For this review, take the finished solid that the model builds, in its own axes (mm). Face numbers are marked on the shaded views. A direction names the side the tool comes from. Round coordinates to 2 decimals unless told otherwise and drop trailing zeros. Loops run counter-clockwise (first coordinate to the right, second up) from the corner with the lowest first, then second, coordinate; pieces in that order, holes last.
1) Wall thickness on L1, parallel to Z at x = -37, y = -20.95; L2, parallel to X at y = -1, z = 53; L3, parallel to Z at x = -10, y = 4: over which ranges is each line inside the solid? List them lowest first.
2) Mouldability with a two-part tool opening along X and no side actions: class the marked faces 6, 7 and 8 as pulls with the +X half, pulls with the -X half, needs draft (parallel to the pull), parting line crosses it, or undercut.
3) Take a section at B-B (z = 60). State the section outline as (x, y) points.
4) Take a section at D-D (x = -30). State the section outline as (y, z) points.
5) Take a section at C-C (x = 0). State the section outline as (y, z) points.
6) Take a section at A-A (x = 37). State the section outline as (y, z) points.
7) Tool access review of the marked faces 1, 2, 3, 4 and 5: name each direction out of +Z, -Z, +X, -X, +Y, -Y from which nothing blocks a thin tool from reaching the whole face with its end or side.
8) Insertion check: pin 1 (4.5 mm diameter, centred on x = -15.5, y = 0, fed in from -Z); pin 2 (2.5 mm diameter, centred on x = 20, z = 61, fed in from +Y); pin 3 (1.5 mm diameter, centred on x = -36.5, z = 30.5, fed in from +Y); pin 4 (8 mm diameter, centred on x = -2, y = 1, fed in from +Z). Each pin has a flat end and moves straight along its axis. Give the tip position at first contact, or say it passes through.
```python
from build123d import *

# Parameters (mm, degrees)
SKETCH3_R                      = 7.25
BOSS_EXTRUDE1_DEPTH            = 5
M3_CLEARANCE_HOLE1_D           = 3.4
M3_CLEARANCE_HOLE1_CSINK_D     = 3.45
M3_CLEARANCE_HOLE1_CSINK_ANGLE = 90
BOSS_EXTRUDE2_DEPTH            = 80
BOSS_EXTRUDE3_DEPTH            = 10
SKETCH16_R                     = 11
CUT_EXTRUDE1_DEPTH             = 7
CUT_EXTRUDE2_REACH             = 90
SKETCH17_R                     = 7
CHAMFER2_SIZE                  = 0.5
CHAMFER3_SIZE                  = 0.5
SKETCH18_W                     = 95
SKETCH18_H                     = 5.838314525
BOSS_EXTRUDE5_DEPTH            = 30
SKETCH21_W                     = 95
SKETCH21_H                     = 5
BOSS_EXTRUDE6_DEPTH            = 30
FILLET1_R                      = 5
M5_CLEARANCE_SLOT1_D           = 5.3


with BuildPart() as part:
    # Sketch3 → Boss-Extrude1 (new body)
    with BuildSketch(Plane.XY):
        with BuildLine():
            Line((22, 0), (22, -22))
            Line((22, -22), (-22, -22))
            Line((-22, -22), (-22, 0))
            ThreePointArc((-22, 0), (0, 22), (22, 0))
        make_face()
        with Locations((0, 7)):
            Circle(SKETCH3_R, mode=Mode.SUBTRACT)
    extrude(amount=BOSS_EXTRUDE1_DEPTH)

    # M3 Clearance Hole1 (through all)
    with Locations(Plane(origin=(0, 0, 0), x_dir=(-1, 0, 0), z_dir=(0, 0, -1))):
        with Locations((-15.5, 0), (15.5, 0), (7.75, 13.423393759), (-7.75, 13.423393759), (-7.75, -13.423393759), (7.75, -13.423393759)):
            CounterSinkHole(M3_CLEARANCE_HOLE1_D / 2, M3_CLEARANCE_HOLE1_CSINK_D / 2, counter_sink_angle=M3_CLEARANCE_HOLE1_CSINK_ANGLE)

    # Sketch7 → Boss-Extrude2 (add)
    with BuildSketch(Plane.XY.offset(5)):
        with BuildLine():
            Line((-19, 0), (-22, 0))
            Line((-22, 0), (-22, -22))
            Line((-22, -22), (22, -22))
            Line((22, -22), (22, 0))
            Line((22, 0), (19, 0))
            ThreePointArc((19, 0), (0, -19), (-19, 0))
        make_face()
    extrude(amount=BOSS_EXTRUDE2_DEPTH)

    # Sketch9 → Boss-Extrude3 (add)
    with BuildSketch(Plane.XY.offset(85)):
        with BuildLine():
            Line((22, 0), (22, -22))
            Line((22, -22), (-22, -22))
            Line((-22, -22), (-22, 0))
            ThreePointArc((-22, 0), (0, 22), (22, 0))
        make_face()
    extrude(amount=BOSS_EXTRUDE3_DEPTH)

    # Sketch16 → Cut-Extrude1 (cut)
    with BuildSketch(Plane.XY.offset(95)):
        with Locations((0, 7)):
            Circle(SKETCH16_R)
    extrude(amount=-CUT_EXTRUDE1_DEPTH, mode=Mode.SUBTRACT)

    # Sketch17 → Cut-Extrude2 (cut, up to next)
    with BuildSketch(Plane.XY.offset(88), mode=Mode.PRIVATE) as cut_extrude2_sk1:
        with Locations((0, 7)):
            Circle(SKETCH17_R)
    cut_extrude2_tool1 = extrude(cut_extrude2_sk1.sketch, amount=-CUT_EXTRUDE2_REACH, mode=Mode.PRIVATE) & part.part
    add(cut_extrude2_tool1.solids().sort_by_distance((0, 7, 88))[0], mode=Mode.SUBTRACT)

    # Chamfer2
    chamfer2_edges = [part.edges().sort_by_distance(p)[0] for p in [
        (-11, 7, 95),
    ]]
    chamfer(chamfer2_edges, length=CHAMFER2_SIZE)

    # Chamfer3
    chamfer3_edges = [part.edges().sort_by_distance(p)[0] for p in [
        (-7.25, 7, 5),
    ]]
    chamfer(chamfer3_edges, length=CHAMFER3_SIZE)

    # Sketch18 → Boss-Extrude5 (add)
    with BuildSketch(Plane(origin=(22, 0, 0), x_dir=(0, 0, -1), z_dir=(1, 0, 0))):
        with Locations((-47.5, -19.080842737)):
            Rectangle(SKETCH18_W, SKETCH18_H)
    extrude(amount=BOSS_EXTRUDE5_DEPTH)

    # Sketch21 → Boss-Extrude6 (add)
    with BuildSketch(Plane.ZY.offset(22)):
        with Locations((47.5, -19.5)):
            Rectangle(SKETCH21_W, SKETCH21_H)
    extrude(amount=BOSS_EXTRUDE6_DEPTH)

    # Fillet1
    fillet1_edges = [part.edges().sort_by_distance(p)[0] for p in [
        (22, -16.161685475, 47.5),
        (-22, -17, 47.5),
    ]]
    fillet(fillet1_edges, radius=FILLET1_R)

    # M5 Clearance Slot1 (through all)
    with Locations(Plane(origin=(0, -22, 0), x_dir=(-1, 0, 0), z_dir=(0, -1, 0))):
        with Locations((37, -80), (-37, -80), (-37, -15), (37, -15)):
            Hole(M5_CLEARANCE_SLOT1_D / 2)


solid = part.part
```
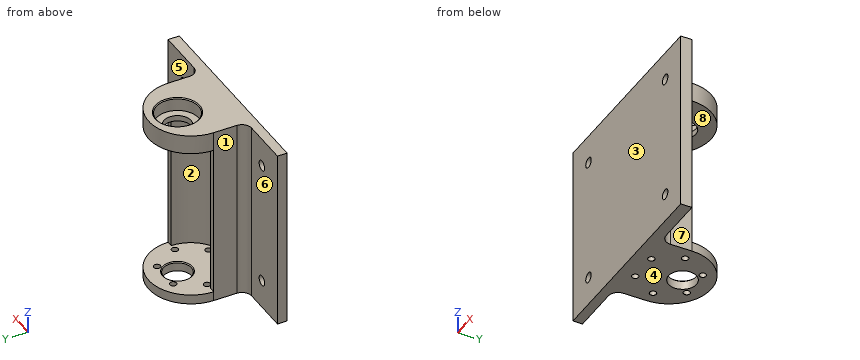
Response:
1. L1: z = 0 to 12.35, 17.65 to 77.35, 82.65 to 95
1. L2: x = -22 to -18.97, 18.97 to 22
1. L3: z = 0 to 5, 85 to 88
2. face 6: needs draft
2. face 7: pulls with the +X half
2. face 8: undercut
3. outline: (-52, -22) - (52, -22) - (52, -16.16) - (27, -16.16) arc R5 cw to (22, -11.16) - (22, 0) - (19, 0) arc R19 cw to (-19, 0) - (-22, 0) - (-22, -12) arc R5 cw to (-27, -17) - (-52, -17) - close
4. outline: (-22, 0) - (-17, 0) - (-17, 95) - (-22, 95) - close
5. outline: (-22, 0) - (-0.25, 0) - (-0.25, 4.5) - (-0.75, 5) - (-19, 5) - (-19, 85) - (0, 85) - (0, 88) - (-4, 88) - (-4, 94.5) - (-4.5, 95) - (-22, 95) - close; (14, 85) - (22, 85) - (22, 95) - (18.5, 95) - (18, 94.5) - (18, 88) - (14, 88) - close; (14.25, 0) - (22, 0) - (22, 5) - (14.75, 5) - (14.25, 4.5) - close
6. outline: (-22, 0) - (-16.16, 0) - (-16.16, 12.35) - (-22, 12.35) - close; (-22, 17.65) - (-16.16, 17.65) - (-16.16, 77.35) - (-22, 77.35) - close; (-22, 82.65) - (-16.16, 82.65) - (-16.16, 95) - (-22, 95) - close
7. face 1: +Z, -Z, -X, +Y
7. face 2: +Y
7. face 3: +Z, -Z, +X, -X, -Y
7. face 4: -Z, +X, -X, +Y, -Y
7. face 5: +Z, -Z, +X, +Y
8. pin 1: stops at z = 0
8. pin 2: stops at y = 0
8. pin 3: stops at y = -17
8. pin 4: stops at z = 88
